For this review, take the finished solid that the model builds, in its own axes (mm). Face numbers are marked on the shaded views. A direction names the side the tool comes from. Give positions to 0.01 mm unless a question says otherwise; leave off trailing zeros. Order: outer loops, then holes, each group sorted by start corner. A loop starts at its lowest first (then second) coordinate and runs counter-clockwise, first axis right, second up.
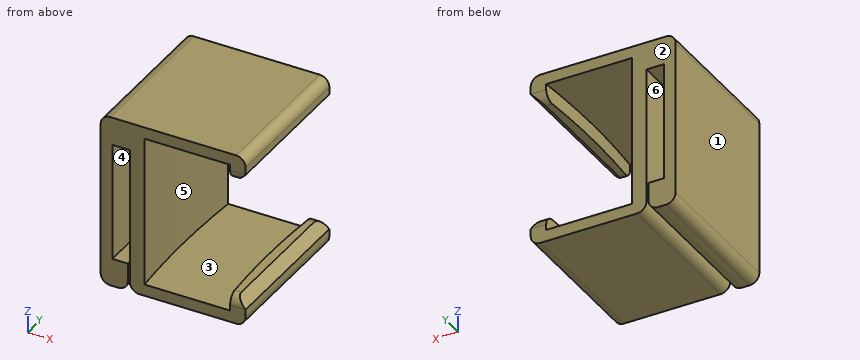
from build123d import *

# Parameters (mm, degrees)
SKETCH032_W     = 11.9495428665
SKETCH032_H     = 15.3649565959
PAD021_DEPTH    = 1.2
PAD022_DEPTH    = 15.6
SKETCH034_W     = 11.9495428665
SKETCH034_H     = 15.3649565959
PAD023_DEPTH    = 1.2
PAD024_DEPTH    = 1.6
PAD025_DEPTH    = 1.6
PAD026_DEPTH    = 15.3649565959
CHAMFER009_SIZE = 1
FILLET003_R     = 1


with BuildPart() as part:
    # Sketch032 → Pad021 (new body)
    with BuildSketch(Plane.XY):
        with Locations((-88.6252285667, 0)):
            Rectangle(SKETCH032_W, SKETCH032_H)
    extrude(amount=PAD021_DEPTH)

    # Sketch033 → Pad022 (join)
    with BuildSketch(Plane.XY.offset(1.2)):
        with BuildLine():
            ThreePointArc((-93.0835083525, 7.682478298), (-93.4, 0), (-93.0835083525, -7.682478298))
            Line((-94.6, -7.682478298), (-93.0835083525, -7.682478298))
            Line((-94.6, 7.682478298), (-94.6, -7.682478298))
            Line((-93.0835083525, 7.682478298), (-94.6, 7.682478298))
        make_face()
    extrude(amount=PAD022_DEPTH)

    # Sketch034 → Pad023 (join)
    with BuildSketch(Plane.XY.offset(16.8)):
        with Locations((-88.6252285667, 0)):
            Rectangle(SKETCH034_W, SKETCH034_H)
    extrude(amount=PAD023_DEPTH)

    # Sketch035 → Pad024 (join)
    with BuildSketch(Plane.XY.offset(1.2)):
        with BuildLine():
            ThreePointArc((-84.2504571335, 7.682478298), (-84.6, 0), (-84.2504571335, -7.682478298))
            Line((-82.6504571335, -7.682478298), (-84.2504571335, -7.682478298))
            Line((-82.6504571335, 7.682478298), (-82.6504571335, -7.682478298))
            Line((-84.2504571335, 7.682478298), (-82.6504571335, 7.682478298))
        make_face()
    extrude(amount=PAD024_DEPTH)

    # Sketch036 → Pad025 (join)
    with BuildSketch(Plane.XY.offset(16.8)):
        with BuildLine():
            ThreePointArc((-84.2504571335, 7.682478298), (-84.6, 0), (-84.2504571335, -7.682478298))
            Line((-82.6504571335, -7.682478298), (-84.2504571335, -7.682478298))
            Line((-82.6504571335, 7.682478298), (-82.6504571335, -7.682478298))
            Line((-84.2504571335, 7.682478298), (-82.6504571335, 7.682478298))
        make_face()
    extrude(amount=-PAD025_DEPTH)

    # Sketch031 (on Plane of DatumPlane) → Pad026 (join)
    with BuildSketch(Plane(origin=(-94.6, -7.682478298, 0), x_dir=(-1, 0, 0), z_dir=(0, 1, 0))):
        Polygon((0, 15.1), (0, 18), (3, 18), (3, 0), (0.2, 0), (0.2, 2.9), (1.8, 2.9), (1.8, 15.1), align=None)
    extrude(amount=PAD026_DEPTH)

    # Chamfer009
    chamfer009_edges = [part.edges().sort_by_distance(p)[0] for p in [
        (-82.650457, 0, 15.2),
        (-82.650457, 0, 2.8),
    ]]
    chamfer(chamfer009_edges, length=CHAMFER009_SIZE)

    # Fillet003
    fillet003_edges = [part.edges().sort_by_distance(p)[0] for p in [
        (-97.6, 0, 0),
        (-97.6, 0, 18),
        (-94.8, 0, 0),
        (-94.6, 0, 0),
        (-82.650457, 0, 0),
        (-83.950457, 7.682478, 2.8),
        (-83.950457, 7.682478, 15.2),
        (-83.950457, -7.682478, 2.8),
        (-83.950457, -7.682478, 15.2),
        (-82.650457, 0, 18),
    ]]
    fillet(fillet003_edges, radius=FILLET003_R)


with BuildPart() as part_1:
    # Body008 placement: moved
    add(part.part.moved(Location((0, 0, -1.4))))


solid = part_1.part
1) Clearance check with flat-ended pins moving along their axes: pin 1 (0.6 mm diameter, centred on y = 1, z = 1, fed in from +X); pin 2 (4 mm diameter, centred on y = -6, z = 8.5, fed in from +X). State where each tip first meets the part, or that it passes through.
Answer sheet:
pin 1: stops at x = -82.95
pin 2: stops at x = -93.08
2) To check wall thickness, follow line 1 (Z direction, x = -84.75, y = 0.5); line 2 (X direction, y = 0, z = 10.75); line 3 (Z direction, x = -83.75, y = 3.25). State the ranges of each line that lie inside material, in increasing order.
Answer sheet:
line 1: z = -1.4 to -0.2, 15.4 to 16.6
line 2: x = -97.6 to -96.4, -94.6 to -93.4
line 3: z = -1.4 to 1.4, 13.8 to 16.6
3) We need section C-C on y = 1.5. Give the boundary of the cut face in (x, z), then the cut area to 3 significant figures.
Answer sheet:
outline: (-97.6, -0.4) arc R1 ccw to (-96.6, -1.4) - (-95.8, -1.4) arc R1 ccw to (-94.8, -0.4) - (-94.8, 1.5) - (-96.4, 1.5) - (-96.4, 13.7) - (-94.6, 13.7) - (-94.6, -0.4) arc R1 ccw to (-93.6, -1.4) - (-83.65, -1.4) arc R1 ccw to (-82.65, -0.4) - (-82.65, 0.4) - (-83.65, 1.4) - (-84.59, 1.4) - (-84.59, -0.2) - (-93.39, -0.2) - (-93.39, 15.4) - (-84.59, 15.4) - (-84.59, 13.8) - (-83.65, 13.8) - (-82.65, 14.8) - (-82.65, 15.6) arc R1 ccw to (-83.65, 16.6) - (-96.6, 16.6) arc R1 ccw to (-97.6, 15.6) - close
area: 83.0 mm2
4) We need section D-D on y = 4.5. Give the boundary of the cut face in (x, z), then the cut area to 3 significant figures.
Answer sheet:
outline: (-97.6, -0.4) arc R1 ccw to (-96.6, -1.4) - (-95.8, -1.4) arc R1 ccw to (-94.8, -0.4) - (-94.8, 1.5) - (-96.4, 1.5) - (-96.4, 13.7) - (-94.6, 13.7) - (-94.6, -0.4) arc R1 ccw to (-93.6, -1.4) - (-83.65, -1.4) arc R1 ccw to (-82.65, -0.4) - (-82.65, 0.4) - (-83.65, 1.4) - (-84.48, 1.4) - (-84.48, -0.2) - (-93.29, -0.2) - (-93.29, 15.4) - (-84.48, 15.4) - (-84.48, 13.8) - (-83.65, 13.8) - (-82.65, 14.8) - (-82.65, 15.6) arc R1 ccw to (-83.65, 16.6) - (-96.6, 16.6) arc R1 ccw to (-97.6, 15.6) - close
area: 84.1 mm2
5) We need section A-A on x = -88.5. Give the boundary of the cut face in (y, z).
Answer sheet:
outline: (-7.68, -1.4) - (7.68, -1.4) - (7.68, -0.2) - (-7.68, -0.2) - close; (-7.68, 15.4) - (7.68, 15.4) - (7.68, 16.6) - (-7.68, 16.6) - close
6) We need section B-B on z = 4.5. Give the boundary of the cut face in (x, y), then the cut area to 3 significant figures.
Answer sheet:
outline: (-97.6, -7.68) - (-96.4, -7.68) - (-96.4, 7.68) - (-97.6, 7.68) - close; (-94.6, -7.68) - (-93.08, -7.68) arc R93.4 cw to (-93.08, 7.68) - (-94.6, 7.68) - close
area: 38.5 mm2
7) Tool access review of the marked faces 4, 5 and 6: name each direction out of +Z, -Z, +X, -X, +Y, -Y from which nothing blocks a thin tool from reaching the whole face with its end or side.
Answer sheet:
face 4: +Y, -Y
face 5: none
face 6: -Z, +Y, -Y
8) Draft analysis for pull direction X (two halves, no side actions). For the marked faces 1, 2 and 3, state which applies: +X half, -X half, draft (parallel to the pull), parting line (faces both ways), or undercut.
Answer sheet:
face 1: -X half
face 2: draft
face 3: undercut
